Build history of the part. All positions in model axes, mm. Face numbers are marked on the shaded views. A direction names the side the tool comes from. Give positions to 0.01 mm unless a question says otherwise; leave off trailing zeros. Order: outer loops, then holes, each group sorted by start corner. A loop starts at its lowest first (then second) coordinate and runs counter-clockwise, first axis right, second up. Notation, with made-up numbers: (18.25, 85) - (52.25, 85) arc R30 cw to (52.25, 120) - close; hole circle Ø4 at (53.5, 23.5). An arc over 180 degrees is marked (long way). Write each question's results on one line, items separated by ' | '. Start each with the question number.
1) Drop flat-ended pins along their axis: pin 1 Ø4 at (y, z) = (2, -52.5) entering from +X; pin 2 Ø8 at (x, z) = (-26.5, -33.5) entering from -Y; pin 3 Ø1.9 at (x, z) = (-37.4, -2.75) entering from -Y. Give the stop position or say it passes through.
2) Drill centre lines: line 1 along Z through (x, y) = (-37.4, -3.4); line 2 along Z through (x, y) = (-22, 1.5); line 3 along Z through (x, y) = (-37.4, -1.9). Where is each one in solid material? Low to high. Write a range as from..to.
3) Tool access for the marked faces 1 and 2: list every direction of +Z, -Z, +X, -X, +Y, -Y with a clear straight run to the whole face (end or side of a thin tool).
4) Cut at B-B on x = -29. List the corners of the cut face in (y, z), plus the area to 3 significant figures.
5) Cut at D-D on y = 1.25. State how many separate pieces and enclosed holes the cut face has, plus the area to 3 significant figures.
6) Two-plate mould, pull along Z, no slides. Class the marked faces 3, 4 and 5: +Z half, -Z half, draft (parallel to the pull), parting line (faces both ways), or undercut.
7) Cut at C-C on z = -26.5. List the corners of the cut face in (x, y), plus the area to 3 significant figures.
8) Cut at A-A on y = -2. List the corners of the cut face in (x, z).
Autodesk Inventor part; units mm, degrees
ref_plane "YZ Plane" through (0, 0, 0) normal (1, 0, 0) x (0, 1, 0)
ref_plane "XZ Plane" through (0, 0, 0) normal (0, 1, 0) x (-1, 0, 0)
ref_plane "XY Plane" through (0, 0, 0) normal (0, 0, 1) x (1, 0, 0)
sketch "Sketch1" plane through (0, 0, 0) normal (0, 1, 0) x (-1, 0, 0)
  line L0 (0, 0) -> (40, 0)
  line L1 (40, 0) -> (40, -60)
  line L2 (40, -60) -> (0, -60)
  line L3 (0, -60) -> (0, 0)
  circle A0 centre (2.6, -2.75) radius 1.27
  circle A1 centre (37.4, -2.75) radius 1.27
  circle A2 centre (37.4, -57.25) radius 1.27
  circle A3 centre (2.6, -57.25) radius 1.27
  dimension "d1" = 40
  dimension "d2" = 60
  dimension "d15" = 2.54
  dimension "d20" = 2.75
  dimension "d21" = 2.6
  dimension "d22" = 2.54
  dimension "d23" = 2.75
  dimension "d24" = 2.6
  dimension "d25" = 2.54
  dimension "d26" = 2.54
  dimension "d27" = 2.75
  dimension "d28" = 2.75
  dimension "d29" = 2.6
  dimension "d30" = 2.6
extrude "Extrusion1" add sketch "Sketch1" along normal blind 3 contours L0 L1 L2 L3 | A0 | A1 | A2 | A3
sketch "Sketch2" plane through (0, 0, 0) normal (0, -1, 0) x (1, 0, 0)
  line L0 (-40, 0) -> (0, 0)
  line L1 (0, -60) -> (-40, -60)
  arc A0 (-5.2, -2.75) -> (-2.6, -5.35) centre (-2.6, -2.75) ccw
  line L2 (0, 0) -> (0, -60)
  arc A1 (-2.6, -54.65) -> (-5.2, -57.25) centre (-2.6, -57.25) ccw
  arc A2 (-34.8, -57.25) -> (-37.4, -54.65) centre (-37.4, -57.25) ccw
  line L3 (-40, -60) -> (-40, 0)
  arc A3 (-37.4, -5.35) -> (-34.8, -2.75) centre (-37.4, -2.75) ccw
  line L4 (-34.8, -57.25) -> (-34.8, -60)
  line L5 (-34.8, -2.75) -> (-34.8, 0)
  line L6 (-5.2, -57.25) -> (-5.2, -60)
  line L7 (-5.2, -2.75) -> (-5.2, 0)
  line L8 (-37.4, -54.65) -> (-40, -54.65)
  line L9 (0, -5.35) -> (-2.6, -5.35)
  line L10 (-37.4, -5.35) -> (-40, -5.35)
  line L11 (-40, -54.65) -> (-37.4, -54.65)
  line L12 (-2.6, -54.65) -> (0, -54.65)
extrude "Extrusion2" add sketch "Sketch2" along normal blind 5 contours L0 L5 A3 L10 L3 | L0 L2 L9 A0 L7 | L8 A2 L4 L1 L3 | L2 L1 L6 A1 L12
sketch "Sketch4" plane through (0, -5, 0) normal (0, -1, 0) x (1, 0, 0)
  arc A0 (-2.6, -54.65) -> (-5.2, -57.25) centre (-2.6, -57.25) ccw
  arc A1 (-34.8, -57.25) -> (-37.4, -54.65) centre (-37.4, -57.25) ccw
  arc A2 (-5.2, -2.75) -> (-2.6, -5.35) centre (-2.6, -2.75) ccw
  arc A3 (-37.4, -5.35) -> (-34.8, -2.75) centre (-37.4, -2.75) ccw
  point P0 (0, 0)
hole "Hole2" at (-2.6, -5, -57.25) at (-37.4, -5, -57.25) at (-2.6, -5, -2.75) at (-37.4, -5, -2.75) direction (0, 1, 0) diameter 3.2 depth 4 tip angle 118
chamfer "Chamfer1" distance 5 angle 45 12 edges at (-1.3, 0, -54.65) (-4.4385, 0, -55.4115) (-5.2, 0, -58.625) (-35.5615, 0, -55.4115) (-34.8, 0, -58.625) (-38.7, 0, -54.65) (-35.5615, 0, -4.5885) (-38.7, 0, -5.35) (-34.8, 0, -1.375) (-1.3, 0, -5.35) (-4.4385, 0, -4.5885) (-5.2, 0, -1.375)
sketch "Sketch5" plane through (0, 0, 0) normal (0, -1, 0) x (1, 0, 0)
  line L0 (-10.2, 0) -> (-10.2, -2.75)
  line L1 (-29.8, 0) -> (-10.2, 0)
  line L2 (-29.8, -2.75) -> (-29.8, 0)
  arc A0 (-37.4, -10.35) -> (-29.8, -2.75) centre (-37.4, -2.75) ccw
  line L3 (-40, -10.35) -> (-37.4, -10.35)
  line L4 (-40, -49.65) -> (-40, -10.35)
  line L5 (-37.4, -49.65) -> (-40, -49.65)
  arc A1 (-29.8, -57.25) -> (-37.4, -49.65) centre (-37.4, -57.25) ccw
  line L6 (-29.8, -60) -> (-29.8, -57.25)
  line L7 (-10.2, -60) -> (-29.8, -60)
  line L8 (-10.2, -57.25) -> (-10.2, -60)
  arc A2 (-2.6, -49.65) -> (-10.2, -57.25) centre (-2.6, -57.25) ccw
  line L9 (0, -49.65) -> (-2.6, -49.65)
  line L10 (0, -10.35) -> (0, -49.65)
  line L11 (-2.6, -10.35) -> (0, -10.35)
  arc A3 (-10.2, -2.75) -> (-2.6, -10.35) centre (-2.6, -2.75) ccw
  line L12 (-12.5, -57.25) -> (-12.5, -57.7)
  line L13 (-13.4861, -57.7) -> (-26.5139, -57.7)
  line L14 (-27.5, -57.7) -> (-27.5, -57.25)
  line L15 (-37.4, -47.35) -> (-37.7, -47.35)
  line L16 (-37.7, -46.3725) -> (-37.7, -13.6275)
  line L17 (-37.7, -12.65) -> (-37.4, -12.65)
  line L18 (-27.5, -2.75) -> (-27.5, -2.3)
  line L19 (-26.5139, -2.3) -> (-13.4861, -2.3)
  line L20 (-12.5, -2.3) -> (-12.5, -2.75)
  line L21 (-2.6, -12.65) -> (-2.3, -12.65)
  line L22 (-2.3, -13.6275) -> (-2.3, -46.3725)
  line L23 (-2.3, -47.35) -> (-2.6, -47.35)
  line L24 (0, -60) -> (-40, -60)
  arc A4 (-5.2, -2.75) -> (-2.6, -5.35) centre (-2.6, -2.75) ccw
  circle A5 centre (-37.4, -2.75) radius 1.6
  line L25 (-0.6615, -56.0122) -> (-2.3, -53.4461)
  line L26 (-4.5385, -58.4878) -> (-5.0416, -57.7)
  line L27 (-34.9584, -57.7) -> (-35.4615, -58.4878)
  line L28 (-37.7, -53.4461) -> (-39.3385, -56.0122)
  arc A6 (-3.2358, -47.3704) -> (-5.1517, -47.6845) centre (-2.6, -57.25) ccw
  arc A7 (-10.2041, -50.9106) -> (-12.4874, -56.7505) centre (-2.6, -57.25) ccw
  arc A8 (-27.5126, -56.7505) -> (-29.7959, -50.9106) centre (-37.4, -57.25) ccw
  arc A9 (-34.8483, -47.6845) -> (-36.7642, -47.3704) centre (-37.4, -57.25) ccw
  arc A10 (-36.7642, -12.6296) -> (-34.8483, -12.3155) centre (-37.4, -2.75) ccw
  arc A11 (-29.7959, -9.0894) -> (-27.5126, -3.2495) centre (-37.4, -2.75) ccw
  arc A12 (-12.4874, -3.2495) -> (-10.2041, -9.0894) centre (-2.6, -2.75) ccw
  arc A13 (-5.1517, -12.3155) -> (-3.2358, -12.6296) centre (-2.6, -2.75) ccw
  line L29 (-6.2523, -47.2565) -> (-16.9275, -30.5382)
  line L30 (-20.8428, -24.4063) -> (-29.8707, -10.2679)
  line L31 (-6.2523, -12.7435) -> (-16.9275, -29.4618)
  line L32 (-20.8428, -35.5937) -> (-29.8707, -49.7321)
  line L33 (-10.1293, -49.7321) -> (-19.1572, -35.5937)
  line L34 (-23.0725, -29.4618) -> (-33.7477, -12.7435)
  line L35 (-10.1293, -10.2679) -> (-19.1572, -24.4063)
  line L36 (-23.0725, -30.5382) -> (-33.7477, -47.2565)
  arc A14 (-3.2358, -47.3704) -> (-2.3, -46.3725) centre (-3.3, -46.3725) ccw
  arc A15 (-6.2523, -47.2565) -> (-5.1517, -47.6845) centre (-5.4095, -46.7183) ccw
  arc A16 (-10.2041, -50.9106) -> (-10.1293, -49.7321) centre (-10.9722, -50.2703) ccw
  arc A17 (-13.4861, -57.7) -> (-12.4874, -56.7505) centre (-13.4861, -56.7) ccw
  arc A18 (-27.5126, -56.7505) -> (-26.5139, -57.7) centre (-26.5139, -56.7) ccw
  arc A19 (-29.8707, -49.7321) -> (-29.7959, -50.9106) centre (-29.0278, -50.2703) ccw
  arc A20 (-34.8483, -47.6845) -> (-33.7477, -47.2565) centre (-34.5905, -46.7183) ccw
  arc A21 (-37.7, -46.3725) -> (-36.7642, -47.3704) centre (-36.7, -46.3725) ccw
  arc A22 (-36.7642, -12.6296) -> (-37.7, -13.6275) centre (-36.7, -13.6275) ccw
  arc A23 (-33.7477, -12.7435) -> (-34.8483, -12.3155) centre (-34.5905, -13.2817) ccw
  arc A24 (-23.0725, -30.5382) -> (-23.0725, -29.4618) centre (-23.9154, -30) ccw
  arc A25 (-19.1572, -35.5937) -> (-20.8428, -35.5937) centre (-20, -36.1318) ccw
  arc A26 (-16.9275, -29.4618) -> (-16.9275, -30.5382) centre (-16.0846, -30) ccw
  arc A27 (-20.8428, -24.4063) -> (-19.1572, -24.4063) centre (-20, -23.8682) ccw
  arc A28 (-5.1517, -12.3155) -> (-6.2523, -12.7435) centre (-5.4095, -13.2817) ccw
  arc A29 (-2.3, -13.6275) -> (-3.2358, -12.6296) centre (-3.3, -13.6275) ccw
  arc A30 (-10.1293, -10.2679) -> (-10.2041, -9.0894) centre (-10.9722, -9.7297) ccw
  arc A31 (-12.4874, -3.2495) -> (-13.4861, -2.3) centre (-13.4861, -3.3) ccw
  arc A32 (-26.5139, -2.3) -> (-27.5126, -3.2495) centre (-26.5139, -3.3) ccw
  arc A33 (-29.7959, -9.0894) -> (-29.8707, -10.2679) centre (-29.0278, -9.7297) ccw
  point P0 (0, 0)
  point P1 (-34.1564, -12.1035)
  point P2 (-30.2793, -9.6279)
  point P3 (-5.8436, -12.1035)
  point P4 (-9.7207, -9.6279)
  point P5 (-5.8436, -47.8965)
  point P6 (-9.7207, -50.3721)
  point P7 (-30.2793, -50.3721)
  point P8 (-34.1564, -47.8965)
  dimension "d57" = 1
extrude "Extrusion3" cut sketch "Sketch5" against normal through all contours L13 A18 A8 A19 L32 A25 L33 A16 A7 A17 | L16 A22 A10 A23 L34 A24 L36 A20 A9 A21 | L19 A31 A12 A30 L35 A27 L30 A33 A11 A32 | L22 A14 A6 A15 L29 A26 L31 A28 A13 A29
fillet "Fillet1" [suppressed]
fillet "Fillet2" radius 2 4 edges at (-40, -1, 0) (-40, -1, -60) (0, -1, -60) (0, -1, 0)
equation "\"d23\" = d20"
equation "\"d24\" = d21"
equation "\"d27\" = d23"
equation "\"d28\" = d20"
equation "\"d29\" = d21"
equation "\"d30\" = d21"
properties part number "Test_PCB_Board_4x6"
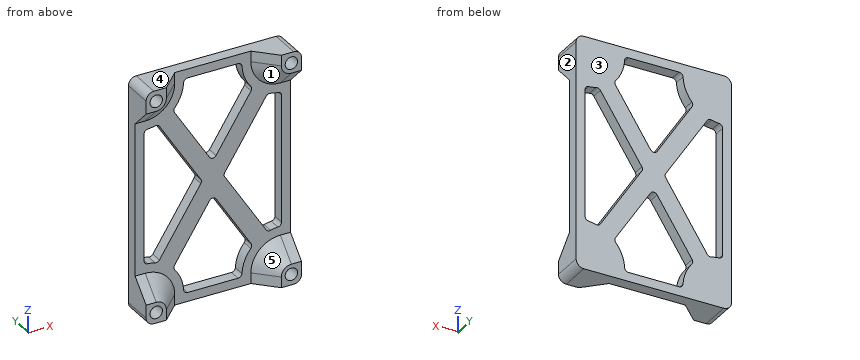
Results:
1) pin 1: x = 0 | pin 2: y = 0 | pin 3: y = -0.61
2) line 1: -60..-58.85, -55.65..-53.05, -6.95..-4.35, -1.15..0 | line 2: -60..-57.7, -37.41..-22.59, -2.3..0 | line 3: -60..-58.85, -55.65..-51.55, -8.45..-4.35, -1.15..0
3) face 1: -Y | face 2: +Z, -Z, +X, +Y, -Y
4) outline: (0, -60) - (3, -60) - (3, -52.01) - (0, -52.01) - close; (0, -48.37) - (3, -48.37) - (3, -39.82) - (0, -39.82) - close; (0, -20.18) - (3, -20.18) - (3, -11.63) - (0, -11.63) - close; (0, -7.99) - (3, -7.99) - (3, 0) - (0, 0) - close | area: 99.2 mm^2
5) separate pieces: 1 | enclosed holes: 4 | area: 1,170 mm^2
6) face 3: draft | face 4: +Z half | face 5: undercut
7) outline: (-40, 0) - (-37.7, 0) - (-37.7, 3) - (-40, 3) - close; (-24.96, 0) - (-15.04, 0) - (-15.04, 3) - (-24.96, 3) - close; (-2.3, 0) - (0, 0) - (0, 3) - (-2.3, 3) - close | area: 43.6 mm^2
8) outline: (-40, -58) arc R2 ccw to (-38, -60) - (-31.8, -60) - (-31.8, -57.25) arc R5.6 ccw to (-37.4, -51.65) - (-40, -51.65) - close; (-40, -8.35) - (-37.4, -8.35) arc R5.6 ccw to (-31.8, -2.75) - (-31.8, 0) - (-38, 0) arc R2 ccw to (-40, -2) - close; (-8.2, -60) - (-2, -60) arc R2 ccw to (0, -58) - (0, -51.65) - (-2.6, -51.65) arc R5.6 ccw to (-8.2, -57.25) - close; (-8.2, -2.75) arc R5.6 ccw to (-2.6, -8.35) - (0, -8.35) - (0, -2) arc R2 ccw to (-2, 0) - (-8.2, 0) - close; hole circle Ø3.2 at (-37.4, -57.25); hole circle Ø3.2 at (-37.4, -2.75); hole circle Ø3.2 at (-2.6, -57.25); hole circle Ø3.2 at (-2.6, -2.75)
